Autodesk Fusion 360 part; units mm, degrees
sketch "スケッチ1" plane through (0, 0, 0) normal (0, 0, 1) x (1, 0, 0)
  line L0 (0, 0) -> (0.238, 0)
  line L1 (0.238, 0) -> (6.238, 0)
  line L2 (6.238, 0) -> (6.238, 4)
  line L3 (0, 0) -> (0, 3)
  line L4 (0, 3) -> (1, 3)
  line L5 (6.238, 4) -> (5.238, 4)
  spline S0 degree 5 poles (1, 3) (1.1004, 3.0037) (1.2998, 3.0125) (1.5949, 3.0299) (1.9802, 3.0617) (2.4472, 3.1166) (2.8983, 3.1882) (3.3319, 3.2779) (3.7472, 3.3868) (4.1446, 3.5143) (4.5253, 3.6593) (4.8176, 3.7881) (5.0303, 3.8915) (5.1692, 3.9633) (5.238, 4) knots 0 0 0 0 0 0 0.1 0.2 0.3 0.4 0.5 0.6 0.7 0.8 0.9 1 1 1 1 1 1
  point P0 (3.4, 3.3)
  dimension "d1" = 6
  dimension "d2" = 4
  dimension "d3" = 3
  dimension "d4" = 1
revolve "回転1" add sketch "スケッチ1" angle 360 about axis through (0, 0, 0) along (0, 1, 0)
sketch "スケッチ2" plane through (0, 0, 0) normal (0, -1, 0) x (1, 0, 0)
  circle A0 centre (0, 0) radius 6.238
  circle A1 centre (0, 0) radius 2.1
  line L0 (0, 0) -> (0, 1.5)
  line L1 (0, 1.5) -> (1.4697, 1.5)
  line L2 (0, 1.5) -> (-1.4697, 1.5)
  line L3 (0, 0) -> (0, -1.5)
  line L4 (0, -1.5) -> (1.4697, -1.5)
  line L5 (0, -1.5) -> (-1.4697, -1.5)
  dimension "d6" = 4.2
  dimension "d7" = 1.5
  dimension "d8" = 1.5
extrude "押し出し1" cut sketch "スケッチ2" against normal blind 2 contours A1 L0 L1 L3 L4 | A1 L0 L2 L3 L5
sketch "スケッチ3" plane through (0, 0, 0) normal (0, -1, 0) x (1, 0, 0)
  line L0 (-1.4697, 1.5) -> (1.4697, 1.5)
  arc A0 (1.4697, -1.5) -> (1.4697, 1.5) centre (0, 0) ccw
  line L1 (1.4697, -1.5) -> (-1.4697, -1.5)
  arc A1 (-1.4697, 1.5) -> (-1.4697, -1.5) centre (0, 0) ccw
  circle A2 centre (0, 0) radius 6.238
  line L2 (0, 1.5) -> (0.2, 1.5)
  line L3 (0, 1.5) -> (-0.2, 1.5)
  line L4 (0, 1.5) -> (0, 1.7)
  line L5 (-0.2, 1.5) -> (0, 1.7)
  line L6 (0, 1.7) -> (0.2, 1.5)
  line L7 (0, -1.5) -> (0.2, -1.5)
  line L8 (0, -1.5) -> (-0.2, -1.5)
  line L9 (0, -1.5) -> (0, -1.7)
  line L10 (0, -1.7) -> (0.2, -1.5)
  line L11 (-0.2, -1.5) -> (0, -1.7)
  dimension "d11" = 0.2
  dimension "d12" = 0.2
  dimension "d13" = 0.2
  dimension "d14" = 0.2
  dimension "d15" = 0.2
  dimension "d16" = 0.2
extrude "押し出し2" cut sketch "スケッチ3" against normal blind 2 contours L0 L3 L4 L5 | L0 L2 L4 L6 | L1 L8 L9 L11 | L1 L7 L9 L10
sketch "スケッチ4" plane through (0, 0, 0) normal (0, -1, 0) x (1, 0, 0)
  line L0 (0, 1.7) -> (0.2, 1.5)
  line L1 (0.2, 1.5) -> (1.4697, 1.5)
  arc A0 (1.4697, -1.5) -> (1.4697, 1.5) centre (0, 0) ccw
  line L2 (1.4697, -1.5) -> (0.2, -1.5)
  line L3 (0.2, -1.5) -> (0, -1.7)
  line L4 (0, -1.7) -> (-0.2, -1.5)
  line L5 (-0.2, -1.5) -> (-1.4697, -1.5)
  arc A1 (-1.4697, 1.5) -> (-1.4697, -1.5) centre (0, 0) ccw
  line L6 (-1.4697, 1.5) -> (-0.2, 1.5)
  line L7 (-0.2, 1.5) -> (0, 1.7)
  circle A2 centre (0, 0) radius 6.238
  line L8 (0, 1.5586) -> (0.1586, 1.4)
  line L9 (0.1586, 1.4) -> (1.4283, 1.4)
  arc A3 (1.4283, -1.4) -> (1.4283, 1.4) centre (0, 0) ccw
  line L10 (1.4283, -1.4) -> (0.1586, -1.4)
  line L11 (0.1586, -1.4) -> (0, -1.5586)
  line L12 (0, -1.5586) -> (-0.1586, -1.4)
  line L13 (-0.1586, -1.4) -> (-1.4283, -1.4)
  arc A4 (-1.4283, 1.4) -> (-1.4283, -1.4) centre (0, 0) ccw
  line L14 (-1.4283, 1.4) -> (-0.1586, 1.4)
  line L15 (-0.1586, 1.4) -> (0, 1.5586)
  dimension "d19" = 0.1
extrude "押し出し3" add sketch "スケッチ4" against normal blind 2 contours L0 L1 A0 L2 L3 L4 L5 A1 L6 L7
extrude "押し出し4" add 1 faces at (0.9388, 0, -3.0134) along direction (0, -1, 0) blind 1
sketch "スケッチ5" plane through (0, -1, 0) normal (0, -1, 0) x (1, 0, 0)
  arc A0 (-1.4283, 1.4) -> (-1.4283, -1.4) centre (0, 0) ccw
  line L0 (-1.4283, 1.4) -> (-0.1586, 1.4)
  line L1 (-0.1586, 1.4) -> (0, 1.5586)
  line L2 (0, 1.5586) -> (0.1586, 1.4)
  line L3 (0.1586, 1.4) -> (1.4283, 1.4)
  arc A1 (1.4283, -1.4) -> (1.4283, 1.4) centre (0, 0) ccw
  line L4 (1.4283, -1.4) -> (0.1586, -1.4)
  line L5 (0.1586, -1.4) -> (0, -1.5586)
  line L6 (0, -1.5586) -> (-0.1586, -1.4)
  line L7 (-0.1586, -1.4) -> (-1.4283, -1.4)
  circle A2 centre (0, 0) radius 6.238
  line L8 (0, 1.7) -> (0.2, 1.5)
  line L9 (0.2, 1.5) -> (1.4697, 1.5)
  arc A3 (1.4697, -1.5) -> (1.4697, 1.5) centre (0, 0) ccw
  line L10 (1.4697, -1.5) -> (0.2, -1.5)
  line L11 (0.2, -1.5) -> (0, -1.7)
  line L12 (0, -1.7) -> (-0.2, -1.5)
  line L13 (-0.2, -1.5) -> (-1.4697, -1.5)
  arc A4 (-1.4697, 1.5) -> (-1.4697, -1.5) centre (0, 0) ccw
  line L14 (-1.4697, 1.5) -> (-0.2, 1.5)
  line L15 (-0.2, 1.5) -> (0, 1.7)
  dimension "d24" = -0.1
extrude "押し出し5" cut sketch "スケッチ5" against normal blind 3 contours L8 L9 A3 L10 L11 L12 L13 A4 L14 L15
sketch "スケッチ6" plane through (0, -1, 0) normal (0, -1, 0) x (1, 0, 0)
  line L0 (-0.2, -1.5) -> (-1.4697, -1.5)
  arc A0 (-1.4697, 1.5) -> (-1.4697, -1.5) centre (0, 0) ccw
  line L1 (-1.4697, 1.5) -> (-0.2, 1.5)
  line L2 (-0.2, 1.5) -> (0, 1.7)
  line L3 (0, 1.7) -> (0.2, 1.5)
  line L4 (0.2, 1.5) -> (1.4697, 1.5)
  arc A1 (1.4697, -1.5) -> (1.4697, 1.5) centre (0, 0) ccw
  line L5 (1.4697, -1.5) -> (0.2, -1.5)
  line L6 (0.2, -1.5) -> (0, -1.7)
  line L7 (0, -1.7) -> (-0.2, -1.5)
  circle A2 centre (0, 0) radius 6.238
  line L8 (-0.1793, -1.45) -> (-1.4491, -1.45)
  arc A3 (-1.4491, 1.45) -> (-1.4491, -1.45) centre (0, 0) ccw
  line L9 (-1.4491, 1.45) -> (-0.1793, 1.45)
  line L10 (-0.1793, 1.45) -> (0, 1.6293)
  line L11 (0, 1.6293) -> (0.1793, 1.45)
  line L12 (0.1793, 1.45) -> (1.4491, 1.45)
  arc A4 (1.4491, -1.45) -> (1.4491, 1.45) centre (0, 0) ccw
  line L13 (1.4491, -1.45) -> (0.1793, -1.45)
  line L14 (0.1793, -1.45) -> (0, -1.6293)
  line L15 (0, -1.6293) -> (-0.1793, -1.45)
  line L16 (-1.4491, 1.45) -> (-1.3991, 1.5)
  line L17 (-1.4491, -1.45) -> (-1.3991, -1.5)
  line L18 (1.4491, -1.45) -> (1.3991, -1.5)
  line L19 (1.4491, 1.45) -> (1.3991, 1.5)
  dimension "d27" = -0.05
extrude "押し出し6" add sketch "スケッチ6" against normal blind 3 contours L0 A0 L1 A3 L16 L17 | L4 A1 L5 A4 L18 L19
For this review, take the finished solid that the model builds, in its own axes (mm). A direction names the side the tool comes from. Coordinates: 2 decimals unless noted, no trailing zeros. Loops run counter-clockwise (first coordinate to the right, second up) from the corner with the lowest first, then second, coordinate; pieces in that order, holes last. Notation, with made-up numbers: (44, 44) - (51, 44) arc R21 ccw to (51, 55) - close; hole circle Ø8 at (85.25, -14.75). An arc over 180 degrees is marked (long way). Use one line per item in the form item = value. Start each with the question number.
1) Draft analysis for pull direction Z (two halves, no side actions). For faces 3 (the face through (-1.35, 1.54, 6.09)), 4 (the face through (-1, 0, -1.5)), 5 (the face through (0, -1, -3)), state which applies: released by +Z, released by -Z, zero draft, split by the parting line, or undercut.
2) For faces 1 (the face through (0, 2, 0)), 2 (the face through (0, 3, 0)), list the 3-axis set-ups (+Z, -Z, +X, -X, +Y, -Y) from which the entire face can be reached by the end or side of a thin tool; tool diameter is ignored.
3) Take a section at A-A (y = 0.25). State the section outline as (x, z) points.
4) For pin 1 (1.3 mm diameter, centred on x = 1, y = 0.5, fed in from -Z); pin 2 (1.5 mm diameter, centred on x = -3.5, y = -0.5, fed in from +Z); pin 3 (1.5 mm diameter, centred on y = 3, z = 3, fed in from -X), all flat-tipped, find the tip position at first contact; note any pin that passes through.
5) To check wall thickness, follow probe 1 along Z at (x, y) = (-0.5, 0.3); probe 2 along Z at (x, y) = (-1.25, 0.5); probe 3 along X at (y, z) = (-0.15, 1). State the ranges of each line that lie inside material, in increasing order. Write a range as from..to.
From the geometry:
q1.face_3 = split by the parting line
q1.face_4 = undercut
q1.face_5 = zero draft
q2.face_1 = -Y
q2.face_2 = +Y
q3.outline = circle Ø12.48 at (0, 0); hole (-1.45, -1.45) - (-1.4, -1.5) - (-0.2, -1.5) - (0, -1.7) - (0.2, -1.5) - (1.4, -1.5) - (1.45, -1.45) arc R2.05 ccw to (1.45, 1.45) - (1.4, 1.5) - (0.2, 1.5) - (0, 1.7) - (-0.2, 1.5) - (-1.4, 1.5) - (-1.45, 1.45) arc R2.05 ccw to start
q4.pin_1 = -6.23
q4.pin_2 = 5.6
q4.pin_3 = -5.82
q5.probe_1 = -6.22..-1.5, 1.5..6.22
q5.probe_2 = -6.11..-1.5, 1.5..6.11
q5.probe_3 = -6.16..-1.79, 1.79..6.16
